Here's how the part is built. I have some questions about the finished solid (model axes, mm). Face numbers are marked on the shaded views. A direction names the side the tool comes from. Give positions to 0.01 mm unless a question says otherwise; leave off trailing zeros. Write each loop counter-clockwise with the first axis right and the second up, starting at its lowest first coordinate (ties: lowest second). Pieces come first, ordered by that corner, then holes. Notation, with made-up numbers: (-3.75, 65.25) -> (19.25, 65.25) arc R22 cw to (19.25, 77.25) -> close; hole circle Ø7 at (71, 22). An arc over 180 degrees is marked (long way). Put each result on its own line as item: value. Start each with the question number.
from build123d import *

# Parameters (mm, degrees)
EXTRUDE_1_DEPTH        = 4
CHAMFER_1_SIZE         = 3
CUT_EXTRUDE_1_DEPTH    = 33.687918257
SKETCH_3_R             = 9.557368967
EXTRUDE_2_DEPTH        = 3
CUT_EXTRUDE_2_DEPTH    = 2
SKETCH_7_R             = 2
CUT_EXTRUDE_3_DEPTH    = 34.188853551
FILLET_2_R             = 1
SKETCH_9_W             = 36
SKETCH_9_H             = 32.5
SKETCH_9_R             = 9.557368967
EXTRUDE_4_DEPTH        = 3
SKETCH_10_W            = 160
SKETCH_10_H            = 85
EXTRUDE_5_DEPTH        = 3
SKETCH_11_W            = 3
SKETCH_11_H            = 85
EXTRUDE_6_DEPTH        = 10
SKETCH_12_W            = 10
SKETCH_12_H            = 6
EXTRUDE_7_DEPTH        = 10
SKETCH_13_W            = 10
SKETCH_13_H            = 10
EXTRUDE_8_DEPTH        = 3
SKETCH_15_W            = 10
SKETCH_15_H            = 16
EXTRUDE_10_DEPTH       = 12.5
SKETCH_17_W            = 10
SKETCH_17_H            = 86
EXTRUDE_11_DEPTH       = 5
CUT_EXTRUDE_5_DEPTH    = 213.052469922
CUT_EXTRUDE_6_DEPTH    = 3
FILLET_3_R             = 5
FILLET_3_OF_MIRROR_2_R = 5
CUT_EXTRUDE_7_DEPTH    = 147.274570586


with BuildPart() as part:
    # 草图1 → 凸台-拉伸1 (new body)
    with BuildSketch(Plane(origin=(0, 0, 0), x_dir=(1, 0, 0), z_dir=(0, 1, 0))):
        Polygon((-8, 28.5), (8, 28.5), (15.5, 0), (-15.5, 0), align=None)
    extrude(amount=EXTRUDE_1_DEPTH)

    # Chamfer 1
    chamfer_1_edges = [part.edges().sort_by_distance(p)[0] for p in [
        (11.75, 4, -14.25),
        (-11.75, 4, -14.25),
    ]]
    chamfer(chamfer_1_edges, length=CHAMFER_1_SIZE)

    # 草图2 → 切除-拉伸1 (cut, through all)
    with BuildSketch(Plane(origin=(0, 4, 0), x_dir=(1, 0, 0), z_dir=(0, 1, 0))):
        Polygon((-4.897860626, 28.5), (-9.315789474, 23.5), (-9.315789474, 28.5), align=None)
        Polygon((9.315789474, 28.5), (4.897860626, 28.5), (9.315789474, 23.5), align=None)
    extrude(amount=-CUT_EXTRUDE_1_DEPTH, mode=Mode.SUBTRACT)

    # 草图3 → 凸台-拉伸2 (add)
    with BuildSketch(Plane(origin=(0, 4, 0), x_dir=(1, 0, 0), z_dir=(0, 1, 0))):
        with Locations(Location((0, 9.557368967, 0), (0, 0, 270))):
            Circle(SKETCH_3_R)
    extrude(amount=EXTRUDE_2_DEPTH)

    # 草图5 → 切除-拉伸2 (cut)
    with BuildSketch(Plane.XZ):
        Polygon((-7.5, -24), (7.5, -24), (7.5, -22), (6, -22), (6, -4), (-6, -4), (-6, -22), (-7.5, -22), align=None)
    extrude(amount=-CUT_EXTRUDE_2_DEPTH, mode=Mode.SUBTRACT)

    # 草图7 → 切除-拉伸3 (cut, through all)
    with BuildSketch(Plane(origin=(0, 7, 0), x_dir=(1, 0, 0), z_dir=(0, 1, 0))):
        with Locations(Location((0, 9.557368967, 0), (0, 0, 270))):
            Circle(SKETCH_7_R)
    extrude(amount=-CUT_EXTRUDE_3_DEPTH, mode=Mode.SUBTRACT)

    # 草图8 → 切除-旋转1 (revolve, cut)
    with BuildSketch(Plane(origin=(0, 0, 0), x_dir=(0, 0, -1), z_dir=(1, 0, 0)), mode=Mode.PRIVATE) as cut_revolve_1_sk:
        Polygon((7.557368967, 5), (5.557368967, 3), (5.557368967, 2), (9.557368967, 2), (9.557368967, 5), align=None)
    revolve(cut_revolve_1_sk.sketch.rotate(Axis((0, -993, -9.557368967), (0, 1, 0)), 180), axis=Axis((0, -993, -9.557368967), (0, 1, 0)), mode=Mode.SUBTRACT)

    # 圆角2
    fillet_2_edges = [part.edges().sort_by_distance(p)[0] for p in [
        (-7.5, 1, -22),
        (-7.5, 1, -24),
        (7.5, 1, -24),
        (7.5, 1, -22),
    ]]
    fillet(fillet_2_edges, radius=FILLET_2_R - 0.0001)  # a hair under: the kernel refuses the full size

    # 草图9 → 凸台-拉伸4 (add)
    with BuildSketch(Plane(origin=(0, 4, 0), x_dir=(1, 0, 0), z_dir=(0, 1, 0))):
        with Locations((0, 12.25)):
            Rectangle(SKETCH_9_W, SKETCH_9_H)
        with Locations((0, 9.557368967)):
            Circle(SKETCH_9_R, mode=Mode.SUBTRACT)
    extrude(amount=EXTRUDE_4_DEPTH)

    # 草图10 → 凸台-拉伸5 (add)
    with BuildSketch(Plane(origin=(0, 7, 0), x_dir=(1, 0, 0), z_dir=(0, 1, 0))):
        with Locations((0, 38.5)):
            Rectangle(SKETCH_10_W, SKETCH_10_H)
    extrude(amount=EXTRUDE_5_DEPTH)

    # 草图11 → 凸台-拉伸6 (add)
    with BuildSketch(Plane(origin=(0, 10, 0), x_dir=(1, 0, 0), z_dir=(0, 1, 0))):
        with Locations((-78.5, 38.5)):
            Rectangle(SKETCH_11_W, SKETCH_11_H)
        with Locations((78.5, 38.5)):
            Rectangle(SKETCH_11_W, SKETCH_11_H)
    extrude(amount=EXTRUDE_6_DEPTH)

    # 草图12 → 凸台-拉伸7 (add)
    with BuildSketch(Plane(origin=(0, 10, 0), x_dir=(1, 0, 0), z_dir=(0, 1, 0))):
        with Locations((-75, 78)):
            Rectangle(SKETCH_12_W, SKETCH_12_H)
        with Locations((75, 78)):
            Rectangle(SKETCH_12_W, SKETCH_12_H)
        with Locations((75, -1)):
            Rectangle(SKETCH_12_W, SKETCH_12_H)
        with Locations((-75, -1)):
            Rectangle(SKETCH_12_W, SKETCH_12_H)
    extrude(amount=EXTRUDE_7_DEPTH)

    # 草图13 → 凸台-拉伸8 (add)
    with BuildSketch(Plane(origin=(0, 20, 0), x_dir=(1, 0, 0), z_dir=(0, 1, 0))):
        with Locations((-75, 76)):
            Rectangle(SKETCH_13_W, SKETCH_13_H)
        with Locations((-75, 1)):
            Rectangle(SKETCH_13_W, SKETCH_13_H)
        with Locations((75, 76)):
            Rectangle(SKETCH_13_W, SKETCH_13_H)
        with Locations((75, 1)):
            Rectangle(SKETCH_13_W, SKETCH_13_H)
    extrude(amount=EXTRUDE_8_DEPTH)

    # 草图15 → 凸台-拉伸10 (add)
    with BuildSketch(Plane.ZY.offset(80)):
        with Locations((-1, 15)):
            Rectangle(SKETCH_15_W, SKETCH_15_H)
    extrude_10 = extrude(amount=EXTRUDE_10_DEPTH)

    # 草图17 → 凸台-拉伸11 (add)
    with BuildSketch(Plane.ZY.offset(92.5)):
        with Locations((-1, 50)):
            Rectangle(SKETCH_17_W, SKETCH_17_H)
    extrude_11 = extrude(amount=EXTRUDE_11_DEPTH)

    # 草图19 → 切除-拉伸5 (cut, symmetric)
    with BuildSketch(Plane(origin=(-92.5, 0, 0), x_dir=(0, 0, -1), z_dir=(1, 0, 0))):
        with BuildLine():
            Line((2.75, 88), (2.75, 28))
            ThreePointArc((2.75, 28), (1, 26.25), (-0.75, 28))
            Line((-0.75, 28), (-0.75, 88))
            ThreePointArc((-0.75, 88), (1, 89.75), (2.75, 88))
        make_face()
    cut_extrude_5 = extrude(amount=CUT_EXTRUDE_5_DEPTH, both=True, mode=Mode.SUBTRACT)

    # 草图20 → 切除-拉伸6 (cut)
    with BuildSketch(Plane.ZY.offset(97.5)):
        with BuildLine():
            Line((2, 88), (2, 28))
            ThreePointArc((2, 28), (-1, 25), (-4, 28))
            Line((-4, 28), (-4, 88))
            ThreePointArc((-4, 88), (-1, 91), (2, 88))
        make_face()
    cut_extrude_6 = extrude(amount=-CUT_EXTRUDE_6_DEPTH, mode=Mode.SUBTRACT)

    # 圆角3
    fillet_3_edges = [part.edges().sort_by_distance(p)[0] for p in [
        (-95, 93, 4),
        (-95, 93, -6),
    ]]
    fillet(fillet_3_edges, radius=FILLET_3_R - 0.0001)  # a hair under: the kernel refuses the full size

    # 镜向2: 凸台-拉伸10, 凸台-拉伸11, 切除-拉伸5, 切除-拉伸6 across plane
    add(extrude_10.mirror(Plane(origin=(0, 0, 0), x_dir=(0, 0, 1), z_dir=(1, 0, 0))))
    add(extrude_11.mirror(Plane(origin=(0, 0, 0), x_dir=(0, 0, 1), z_dir=(1, 0, 0))))
    add(cut_extrude_5.mirror(Plane(origin=(0, 0, 0), x_dir=(0, 0, 1), z_dir=(1, 0, 0))), mode=Mode.SUBTRACT)
    add(cut_extrude_6.mirror(Plane(origin=(0, 0, 0), x_dir=(0, 0, 1), z_dir=(1, 0, 0))), mode=Mode.SUBTRACT)

    # 圆角3 of 镜向2
    fillet_3_of_mirror_2_edges = [part.edges().sort_by_distance(p)[0] for p in [
        (95, 93, 4),
        (95, 93, -6),
    ]]
    fillet(fillet_3_of_mirror_2_edges, radius=FILLET_3_OF_MIRROR_2_R - 0.0001)  # a hair under: the kernel refuses the full size

    # 草图21 → 切除-拉伸7 (cut, through all)
    with BuildSketch(Plane(origin=(0, 20, 0), x_dir=(1, 0, 0), z_dir=(0, 1, 0))):
        Polygon((-65, 81), (65, 81), (0, 48.5), align=None)
        Polygon((-80, 66), (-15, 33.5), (-15, 11), (-80, 11), align=None)
        Polygon((15, 11), (80, 11), (80, 66), (15, 33.5), align=None)
    extrude(amount=-CUT_EXTRUDE_7_DEPTH, mode=Mode.SUBTRACT)


solid = part.part
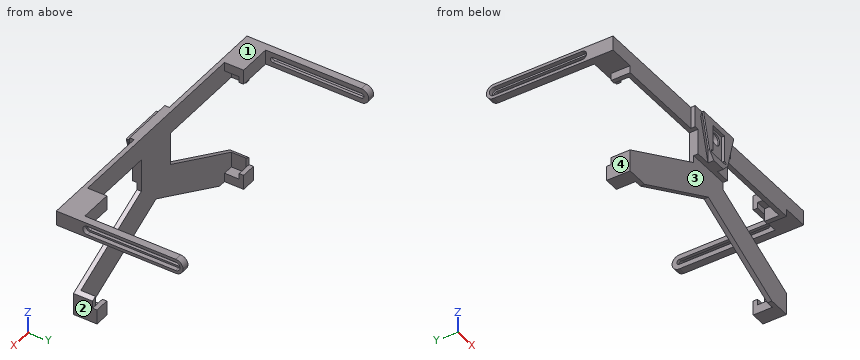
1) I want a section at B-B, the plane z = -53.5. Write out the boundary of the cut face in (x, y).
2) I want a section at C-C, the plane x = 61. Write out the boundary of the cut face in (y, z), and give its area (4 significant figures).
3) Which directions (+Z, -Z, +X, -X, +Y, -Y) give clear straight access to the entire face, cutting with the end or side of a thin tool? Please do the marked faces 1, 2, 3 and 4.
4) I need wall thicknesses on probe 1 along X at (y, z) = (18, -8); probe 2 along Y at (x, z) = (44.5, -51); probe 3 along Z at (x, y) = (-78, 9). Which ranges of each line are inside material? Lowest first, please.
5) I want a section at A-A, the plane y = 55.5. Write out the boundary of the cut face in (x, z).
6) I'm going to push flat-ended pins straight in: pin 1 Ø1.2 at (x, z) = (-72.5, -4.5) entering from -Y; pin 2 Ø3 at (y, z) = (16.5, -75.5) entering from +X; pin 3 Ø3 at (y, z) = (6, -26) entering from +X. Where does each tip first touch, or does it pass through?
Established:
1. outline: (-55, 7) -> (-10, 7) -> (-10, 10) -> (-55, 10) -> close; (10, 7) -> (55, 7) -> (55, 10) -> (10, 10) -> close
2. outline: (7, -79) -> (10, -79) -> (10, -56.5) -> (7, -56.5) -> close; (7, -11) -> (10, -11) -> (10, 4) -> (7, 4) -> close
2. area: 112.5 mm2
3. face 1: +Z, +X, -X, +Y, -Y
3. face 2: -Z, +X, +Y, -Y
3. face 3: -Z, +X, -X, -Y
3. face 4: -Z, -X, +Y, -Y
4. probe 1: x = -80 to -77, 77 to 80
4. probe 2: y = 7 to 10
4. probe 3: z = -81 to -65, -11 to 4
5. outline: (-97.5, -6) -> (-92.5, -6) -> (-92.5, -2.75) -> (-94.5, -2.75) -> (-94.5, -4) -> (-97.5, -4) -> close; (-97.5, 2) -> (-94.5, 2) -> (-94.5, 0.75) -> (-92.5, 0.75) -> (-92.5, 4) -> (-97.5, 4) -> close; (92.5, -6) -> (97.5, -6) -> (97.5, -4) -> (94.5, -4) -> (94.5, -2.75) -> (92.5, -2.75) -> close; (92.5, 0.75) -> (94.5, 0.75) -> (94.5, 2) -> (97.5, 2) -> (97.5, 4) -> (92.5, 4) -> close
6. pin 1: stops at y = 7
6. pin 2: stops at x = 80
6. pin 3: stops at x = 15
